Geometry: final body of the model. Coordinates: model frame, mm. Face numbers are marked on the shaded views. A direction names the side the tool comes from. Coordinates: 2 decimals unless noted, no trailing zeros. Loops run counter-clockwise (first coordinate to the right, second up) from the corner with the lowest first, then second, coordinate; pieces in that order, holes last. Notation, with made-up numbers: (63, 16.5) -> (121, 16.5) arc R11 cw to (121, 35.5) -> close; hole circle Ø10 at (1, 2.25). An arc over 180 degrees is marked (long way). One line per item, written item: value. Start each with the question number.
Item 1: Ray query, probe 1 along X at (y, z) = (-21.5, 30); probe 2 along X at (y, z) = (-8, 17); probe 3 along X at (y, z) = (-14, 30). Return the intervals inside material, ascending. Write a range as from..to.
Item 2: Section query A-A on x = -60. Return loops of the section in (y, z).
Item 3: Set-up query: the marked faces 4 and 5. Return all of +Z, -Z, +X, -X, +Y, -Y with unobstructed straight access to the full face (end or side cutting, diameter ignored); none if empty.
Item 4: Section query C-C on x = -75. Return loops of the section in (y, z), then the cut area to 3 significant figures.
Item 5: Mould query, pull axis X, two halves, no side actions, for the marked faces 1, 2 and 3. Classes: +X half, -X half, draft (parallel to the pull), parting line (faces both ways), or undercut.
Item 6: Section query B-B on z = 21.5. Give the number of separate pieces and of enclosed holes in the cut face, then the cut area to 3 significant figures.
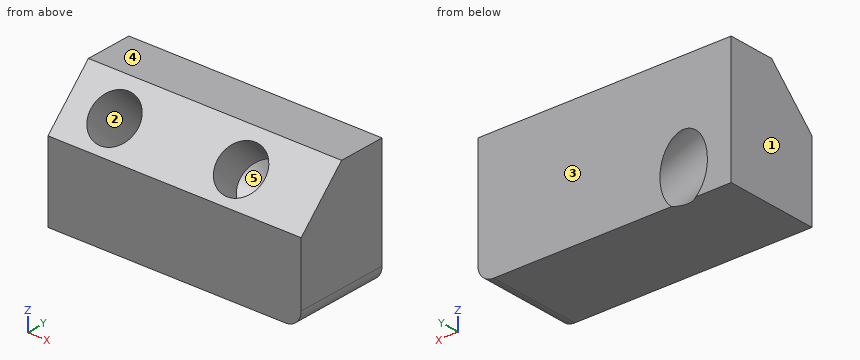
from build123d import *

# Parameters (mm, degrees)
F0_W     = 80
F0_H     = 30
F1_DEPTH = 40
F2_SIZE  = 15
F4_D     = 15
F6_D     = 15
F6_DEPTH = 12
F6_TIP   = 4.5064546427
F7_R     = 5


with BuildPart() as f1:
    # F0 (on Top) → F1 (new body)
    with BuildSketch(Plane.XY):
        with Locations((-40, -15)):
            Rectangle(F0_W, F0_H)
    extrude(amount=F1_DEPTH)

    # F2
    f2_edges = [f1.edges().sort_by_distance(p)[0] for p in [
        (-40, -30, 40),
    ]]
    chamfer(f2_edges, length=F2_SIZE)

    # F4 (through all)
    with Locations(Plane(origin=(0, -27.5, 27.5), x_dir=(1, 0, 0), z_dir=(0, -0.7071067812, 0.7071067812))):
        with Locations((-65, 6.4644660941)):
            Hole(F4_D / 2)

    # F6
    with Locations(Plane(origin=(0, -27.5, 27.5), x_dir=(1, 0, 0), z_dir=(0, -0.7071067812, 0.7071067812))):
        with Locations((-24.9926396036, 6.4644660941)):
            Hole(F6_D / 2, depth=F6_DEPTH)
            with Locations((0, 0, -(F6_DEPTH + F6_TIP / 2))):  # 118° drill point
                Cone(0, F6_D / 2, F6_TIP, mode=Mode.SUBTRACT)

    # F7
    f7_edges = [f1.edges().sort_by_distance(p)[0] for p in [
        (0, -15, 0),
    ]]
    fillet(f7_edges, radius=F7_R)


solid = f1.part
Reply:
1. probe 1: x = -80..-72.49, -57.51..-32.48, -17.51..0
1. probe 2: x = -80..-72.5, -57.5..0
1. probe 3: x = -80..-70.72, -59.28..-30.71, -19.27..0
2. outline: (-30, 0) -> (0, 0) -> (0, 1.24) -> (-26.88, 28.12) -> (-30, 25) -> close; (-18.98, 36.02) -> (0, 17.05) -> (0, 40) -> (-15, 40) -> close
3. face 4: +Z, +X, -X, +Y, -Y
3. face 5: none
4. outline: (-30, 0) -> (0, 0) -> (0, 40) -> (-15, 40) -> (-30, 25) -> close
4. area: 1,090 mm²
5. face 1: -X half
5. face 2: undercut
5. face 3: draft
6. separate pieces: 1
6. enclosed holes: 2
6. area: 2,040 mm²
